Check sheet for the modelled part. Datum: model origin and axes. Units: mm. A direction names the side the tool comes from. Round coordinates to 2 decimals unless told otherwise and drop trailing zeros. Loops run counter-clockwise (first coordinate to the right, second up) from the corner with the lowest first, then second, coordinate; pieces in that order, holes last. Notation, with made-up numbers: (44, 34.5) - (87, 34.5) arc R15 ccw to (87, 38.5) - close; hole circle Ø7 at (83.25, 9). An arc over 180 degrees is marked (long way). Put each result on its own line as item: value.
```python
from build123d import *

# Parameters (mm, degrees)
SKETCH2_W                      = 30
SKETCH2_H                      = 15
BOSS_EXTRUDE1_DEPTH            = 6
CBORE_FOR_M4_SHCS1_D           = 4.8
CBORE_FOR_M4_SHCS1_CBORE_D     = 8
CBORE_FOR_M4_SHCS1_CBORE_DEPTH = 4
BOSS_EXTRUDE2_DEPTH            = 30
CUT_EXTRUDE1_START             = -15
SKETCH6_W                      = 6
SKETCH6_H                      = 18.030958188
SKETCH6_W_2                    = 16.282501636
SKETCH6_H_2                    = 17.921679654
SKETCH6_W_3                    = 7
SKETCH6_H_3                    = 20.435085946
CUT_EXTRUDE1_DEPTH             = 28.107006543
CUT_EXTRUDE2_DEPTH             = 30.966648128
CUT_EXTRUDE2_DEPTH_BACK        = 30.966648128
SKETCH7_R                      = 1.7
FILLET1_R                      = 4


with BuildPart() as part:
    # Sketch2 → Boss-Extrude1 (new body)
    with BuildSketch(Plane.XY):
        with Locations((15, 7.5)):
            Rectangle(SKETCH2_W, SKETCH2_H)
    extrude(amount=BOSS_EXTRUDE1_DEPTH)

    # CBORE for M4 SHCS1 (through all)
    with Locations(Plane.XY.offset(6)):
        with Locations((7.5, 7.5), (22.5, 7.5)):
            CounterBoreHole(CBORE_FOR_M4_SHCS1_D / 2, CBORE_FOR_M4_SHCS1_CBORE_D / 2, CBORE_FOR_M4_SHCS1_CBORE_DEPTH)

    # Sketch5 → Boss-Extrude2 (add)
    with BuildSketch(Plane(origin=(30, 0, 0), x_dir=(0, 0, -1), z_dir=(1, 0, 0))):
        with BuildLine():
            Line((0, 0), (-2, -7))
            ThreePointArc((-2, -7), (-9.236067977, -11.472135955), (-10, -3))
            Line((-10, -3), (-6, 0))
            Line((-6, 0), (0, 0))
        make_face()
    extrude(amount=-BOSS_EXTRUDE2_DEPTH)

    # Sketch6 → Cut-Extrude1 (cut, through all)
    with BuildSketch(Plane(origin=(0, 15, 0), x_dir=(1, 0, 0), z_dir=(0, 1, 0)).offset(CUT_EXTRUDE1_START)):
        with Locations((15, -4.71597722)):
            Rectangle(SKETCH6_W, SKETCH6_H)
        with Locations((-1.141250818, -5.644844763)):
            Rectangle(SKETCH6_W_2, SKETCH6_H_2)
        with Locations((26.5, -5.918041099)):
            Rectangle(SKETCH6_W_3, SKETCH6_H_3)
    extrude(amount=-CUT_EXTRUDE1_DEPTH, mode=Mode.SUBTRACT)

    # Sketch7 → Cut-Extrude2 (cut, two sides: drawn at the far end of the back side and taken through both)
    with BuildSketch(Plane.ZY.offset(-7).offset(-CUT_EXTRUDE2_DEPTH_BACK)):
        with Locations((7, -7)):
            Circle(SKETCH7_R)
    extrude(amount=CUT_EXTRUDE2_DEPTH + CUT_EXTRUDE2_DEPTH_BACK, mode=Mode.SUBTRACT)

    # Fillet1
    # the kernel refuses this fillet: 4 mm, written as the material it takes off along each edge
    with BuildSketch(Plane(origin=(26, 11, 2), x_dir=(0, 0, 1), z_dir=(1, 0, 0))) as fillet1_piece_1_section:
        Polygon((0, 0), (FILLET1_R, 0), (FILLET1_R, -FILLET1_R), (0, -FILLET1_R), align=None)
    fillet1_piece_1 = extrude(amount=FILLET1_R, mode=Mode.PRIVATE)
    fillet1_piece_1 = fillet1_piece_1 - Plane(origin=(26, 11, 2), x_dir=(0, -0.7071067811865475, -0.7071067811865475), z_dir=(1, 0, 0)) * Sphere(FILLET1_R, mode=Mode.PRIVATE)
    add(fillet1_piece_1, mode=Mode.SUBTRACT)
    with BuildSketch(Plane(origin=(4, 11, 2), x_dir=(0, 0, 1), z_dir=(-1, 0, 0))) as fillet1_piece_2_section:
        Polygon((0, 0), (FILLET1_R, 0), (FILLET1_R, FILLET1_R), (0, FILLET1_R), align=None)
    fillet1_piece_2 = extrude(amount=FILLET1_R, mode=Mode.PRIVATE)
    fillet1_piece_2 = fillet1_piece_2 - Plane(origin=(4, 11, 2), x_dir=(0, -0.7071067811865475, -0.7071067811865475), z_dir=(-1, 0, 0)) * Sphere(FILLET1_R, mode=Mode.PRIVATE)
    add(fillet1_piece_2, mode=Mode.SUBTRACT)
    with BuildSketch(Plane(origin=(30, -10, 6), x_dir=(-1, 0, 0), z_dir=(0, 1, 0))) as fillet1_piece_3:
        with BuildLine():
            CenterArc((FILLET1_R, -FILLET1_R), FILLET1_R, 90, 90)
            Line((0, -FILLET1_R), (0, 0))
            Line((0, 0), (FILLET1_R, 0))
        make_face()
    extrude(amount=21, mode=Mode.SUBTRACT)
    with BuildSketch(Plane(origin=(26, 15, 6), x_dir=(0, -1, 0), z_dir=(-1, 0, 0))) as fillet1_piece_4:
        with BuildLine():
            CenterArc((FILLET1_R, -FILLET1_R), FILLET1_R, 90, 90)
            Line((0, -FILLET1_R), (0, 0))
            Line((0, 0), (FILLET1_R, 0))
        make_face()
    extrude(amount=22, mode=Mode.SUBTRACT)
    with BuildSketch(Plane(origin=(0, 11, 6), x_dir=(0, 0, -1), z_dir=(0, -1, 0))) as fillet1_piece_5:
        with BuildLine():
            CenterArc((FILLET1_R, FILLET1_R), FILLET1_R, 180, 90)
            Line((0, FILLET1_R), (0, 0))
            Line((0, 0), (FILLET1_R, 0))
        make_face()
    extrude(amount=21, mode=Mode.SUBTRACT)
    with BuildSketch(Plane(origin=(0, 15, -10), x_dir=(0, -1, 0), z_dir=(0, 0, 1)), Plane(origin=(30, 15, -10), x_dir=(-1, 0, 0), z_dir=(0, 0, 1))) as fillet1_piece_6:
        with BuildLine():
            CenterArc((FILLET1_R, FILLET1_R), FILLET1_R, 180, 90)
            Line((0, FILLET1_R), (0, 0))
            Line((0, 0), (FILLET1_R, 0))
        make_face()
    extrude(amount=12, mode=Mode.SUBTRACT)


solid = part.part
```
Item 1: Section check B-B on y = -10. Enter the section's corners in (x, z).
Filled sheet:
outline: (7, 3) - (12, 3) - (12, 11) - (7, 11) - close; (18, 3) - (23, 3) - (23, 11) - (18, 11) - close
Item 2: Section check A-A on x = 22.5. Enter the section's corners in (y, z), then the cut area to 3 significant figures.
Filled sheet:
outline: (-7, 2) - (0, 0) - (5.1, 0) - (5.1, 2) - (3.5, 2) - (3.5, 6) - (0, 6) - (-3, 10) arc R5 ccw (long way) to start; (9.9, 0) - (15, 0) - (15, 2) arc R4 ccw to (11.5, 5.97) - (11.5, 2) - (9.9, 2) - close; hole circle Ø3.4 at (-7, 7)
area: 138 mm²
Item 3: Section check D-D on x = 19. Enter the section's corners in (y, z).
Filled sheet:
outline: (-7, 2) - (0, 0) - (15, 0) - (15, 2) arc R4 ccw to (11, 6) - (9.44, 6) - (9.44, 2) - (5.56, 2) - (5.56, 6) - (0, 6) - (-3, 10) arc R5 ccw (long way) to start; hole circle Ø3.4 at (-7, 7)
Item 4: Section check C-C on z = 7. Enter the section's corners in (x, y).
Filled sheet:
outline: (7, -12) - (12, -12) - (12, -8.7) - (7, -8.7) - close; (7, -5.3) - (12, -5.3) - (12, -0.75) - (7, -0.75) - close; (18, -12) - (23, -12) - (23, -8.7) - (18, -8.7) - close; (18, -5.3) - (23, -5.3) - (23, -0.75) - (18, -0.75) - close
Item 5: Go/stop test with flat-tipped pins: pin 1 (5 mm diameter, centred on y = 6.5, z = 5, fed in from +X); pin 2 (2.5 mm diameter, centred on x = 9, y = 9.5, fed in from +Z); pin 3 (0.8 mm diameter, centred on x = 25.5, y = 10, fed in from +Z). Record where each tip stops, or that it passes through.
Filled sheet:
pin 1: x = 29.97
pin 2: z = 2
pin 3: z = 6
Item 6: Thickness scan on line 1 (X direction, y = -10.5, z = 10.5); line 2 (X direction, y = 5, z = 2.75); line 3 (X direction, y = 10.25, z = 5). Record the ranges inside material, lowest first. Write a range as from..to.
Filled sheet:
line 1: 7..12, 18..23
line 2: 0.07..4.38, 10.62..19.38, 25.62..29.93
line 3: 1.35..4.6, 10.4..19.6, 25.4..28.65
Item 7: Release check for a two-part mould opening along X. For faces 4 (the flat face through (15, 0, 3)), 5 (the flat face through (22.4, 4.9, 2)), 6 (the cylindrical face through (1.203, 5.577, 4.859)), 7 (the flat face through (26, 0, 3)) record: +X half, -X half, draft (parallel to the pull), parting line (faces both ways), or undercut.
Filled sheet:
face 4: undercut
face 5: undercut
face 6: -X half
face 7: draft
Item 8: Tool access check on faces 1 (the cylindrical face through (6.633, 3.595, 4.028)), 2 (the flat face through (25.6, 10.6, 6)), 3 (the flat face through (3, 0, 3)). Record the directions out of +Z, -Z, +X, -X, +Y, -Y that give a thin tool (end or side, any length) a straight path to the whole face; none if there is none.
Filled sheet:
face 1: +Z
face 2: +Z, +X, -X, +Y, -Y
face 3: +Z, -Z, -X, -Y
